Work out the finished part from the listing and answer in its coordinate system (mm). A direction names the side the tool comes from. Round coordinates to 2 decimals unless told otherwise and drop trailing zeros. Order: outer loops, then holes, each group sorted by start corner. A loop starts at its lowest first (then second) coordinate and runs counter-clockwise, first axis right, second up. Notation, with made-up numbers: M -33.5,-27.75 L 19.5,-27.75 A13 ccw 19.5,-12.75 Z; hole C -17.5,59 d5. An arc over 180 degrees is marked long. Return JSON: item names as keys, results as strings.
from build123d import *

# Parameters (mm, degrees)
BOSS_EXTRUDE3_DEPTH    = 50.8
SKETCH8_R              = 6
PANEL_MOUNT_HOLE_DEPTH = 4
CUT_EXTRUDE1_REACH     = 5.18
SKETCH9_R              = 3.96875


with BuildPart() as part:
    # Sketch1 → Boss-Extrude3 (new body)
    with BuildSketch(Plane(origin=(0, 0, 0), x_dir=(1, 0, 0), z_dir=(0, 1, 0))):
        Polygon((-19.05, 63.5), (-19.05, 60.325), (-3.175, 60.325), (-3.175, 3.18), (-19.05, 3.18), (-19.05, 0), (0, 0), (0, 63.5), align=None)
    extrude(amount=BOSS_EXTRUDE3_DEPTH)

    # Sketch8 → Panel Mount Hole (cut)
    with BuildSketch(Plane(origin=(0, 0, -63.5), x_dir=(-1, 0, 0), z_dir=(0, 0, -1))):
        with Locations((11.2, 36.5125)):
            Circle(SKETCH8_R)
    extrude(amount=-PANEL_MOUNT_HOLE_DEPTH, mode=Mode.SUBTRACT)

    # Sketch9 → Cut-Extrude1 (cut, up to next)
    with BuildSketch(Plane(origin=(0, 0, -3.18), x_dir=(-1, 0, 0), z_dir=(0, 0, -1)), mode=Mode.PRIVATE) as cut_extrude1_sk1:
        with Locations((13.335, 36.5125)):
            Circle(SKETCH9_R)
    cut_extrude1_tool1 = extrude(cut_extrude1_sk1.sketch, amount=-CUT_EXTRUDE1_REACH, mode=Mode.PRIVATE) & part.part
    add(cut_extrude1_tool1.solids().sort_by_distance((-13.335, 36.5125, -3.18))[0], mode=Mode.SUBTRACT)
    # Sketch9 → Cut-Extrude1 (cut, up to next)
    with BuildSketch(Plane(origin=(0, 0, -3.18), x_dir=(-1, 0, 0), z_dir=(0, 0, -1)), mode=Mode.PRIVATE) as cut_extrude1_sk2:
        with Locations((13.335, 11.1125)):
            Circle(SKETCH9_R)
    cut_extrude1_tool2 = extrude(cut_extrude1_sk2.sketch, amount=-CUT_EXTRUDE1_REACH, mode=Mode.PRIVATE) & part.part
    add(cut_extrude1_tool2.solids().sort_by_distance((-13.335, 11.1125, -3.18))[0], mode=Mode.SUBTRACT)


solid = part.part
Item 1: Each of these flat-tipped pins is pushed along its axis until it touches: pin 1 (2 mm diameter, centred on x = -4.5, z = -23, fed in from +Y); pin 2 (4 mm diameter, centred on y = 23, z = -18, fed in from -X) (3 decimals). Where does it stop, or does it pass through?
Output:
{"pin 1": "passes through", "pin 2": "stops at x = -3.175"}
Item 2: Consider line 1 along Z through (x, y) = (-10.75, 29) (3 decimals); line 2 along Y through (x, z) = (-11.2, -61.2); line 3 along X through (y, z) = (41, -3.5) (3 decimals). Determine where each line is inside the solid, lowest interval first. Write a range as [from, to].
Output:
{"line 1": "z = [-63.5, -60.325], [-3.18, 0]", "line 2": "y = [0, 30.51], [42.51, 50.8]", "line 3": "x = [-3.175, 0]"}
Item 3: Find section D-D (z = -31). Determine the outline of the cut face in (x, y) (3 decimals).
Output:
{"outline": "M -3.175,0 L 0,0 L 0,50.8 L -3.175,50.8 Z"}
Item 4: The mould has two halves that part along Y. Classify faces 1 (the flat face through (-3, 50.8, -30)), 2 (the cylindrical face through (-17, 9.59, -1.61)), 3 (the flat face through (-19.05, 25, -2)), 4 (the cylindrical face through (-15.47, 39.86, -1.61)): pulls with the +Y half, pulls with the -Y half, needs draft (parallel to the pull), parting line crosses it, or undercut.
Output:
{"face 1": "pulls with the +Y half", "face 2": "undercut", "face 3": "needs draft", "face 4": "undercut"}
Item 5: Find section B-B (x = -15.5). Determine the outline of the cut face in (y, z) (3 decimals).
Output:
{"outline": "M 0,-63.5 L 32.328,-63.5 L 32.328,-60.325 L 0,-60.325 Z; M 0,-3.18 L 7.786,-3.18 L 7.786,0 L 0,0 Z; M 14.439,-3.18 L 33.186,-3.18 L 33.186,0 L 14.439,0 Z; M 39.839,-3.18 L 50.8,-3.18 L 50.8,0 L 39.839,0 Z; M 40.697,-63.5 L 50.8,-63.5 L 50.8,-60.325 L 40.697,-60.325 Z"}
Item 6: Find section C-C (y = 17.5). Determine the outline of the cut face in (x, z) (3 decimals).
Output:
{"outline": "M -19.05,-63.5 L 0,-63.5 L 0,0 L -19.05,0 L -19.05,-3.18 L -3.175,-3.18 L -3.175,-60.325 L -19.05,-60.325 Z"}
Item 7: Which of the six approach directions +Z, -Z, +X, -X, +Y, -Y give full straight-line access (tool end or side, diameter ignored) to faces 5 (the flat face through (-11, 25, -60.325)), 6 (the flat face through (-3, 0, -30)), 7 (the cylindrical face through (-9.899, 30.655, -61.935))?
Output:
{"face 5": "-X, +Y, -Y", "face 6": "+Z, -Z, +X, -X, -Y", "face 7": "-Z"}
Item 8: Find section A-A (x = -4.25). Determine the outline of the cut face in (y, z) (3 decimals), plus the area to 3 significant figures.
Output:
{"outline": "M 0,-63.5 L 50.8,-63.5 L 50.8,-60.325 L 0,-60.325 Z; M 0,-3.18 L 50.8,-3.18 L 50.8,0 L 0,0 Z", "area": "323 mm^2"}
